Input: part model. Units: mm. Frame: model coordinates. A direction names the side the tool comes from. Coordinates: 2 decimals unless noted, no trailing zeros. Write each loop counter-clockwise with the first axis right and the second up, starting at its lowest first coordinate (ties: lowest second). Pieces come first, ordered by that corner, then holes. Notation, with made-up numbers: (79.25, 33.25) - (83.25, 33.25) arc R22 cw to (83.25, 57.25) - close; hole circle Ø11 at (16, -33). An arc over 180 degrees is marked (long way). Use a Markdown table: item, result. Add a question column.
Q1. Mould query, pull axis X, two halves, no side actions, for faces 4 (the face through (-20.63, -15.53, 2.46)), 5 (the face through (1, 36.091, 2)), 6 (the face through (-27.03, 12.79, 2.46)). Classes: released by +X, released by -X, zero draft, split by the parting line, or undercut.
Q2. Section query A-A (x = 0). Return the cut outline in (y, z).
Q3. Material intervals for probe 1 along Y at (x, z) = (0, 4); probe 2 along X at (y, z) = (-17, 2.2); probe 3 along X at (y, z) = (2.5, 2.65), sorted ascending. Write a range as from..to.
Q4. Set-up query: faces 1 (the face through (26.8, -5.44, 2.46)), 2 (the face through (19.285, -16.785, 2.465)), 3 (the face through (-27.802, -2.365, 2.465)). Return all of +Z, -Z, +X, -X, +Y, -Y with unobstructed straight access to the full face (end or side cutting, diameter ignored); none if empty.
Q5. Section query C-C (x = -10.5). Return the cut outline in (y, z), then the cut area to 3 significant figures.
Q6. Section query B-B (y = 1). Return the cut outline in (x, z), then the cut area to 3 significant figures.
Q7. Pin query (flat end, axial travel): P1, Ø1, axis at y = 4, z = 1.5, coming from the +X side; P2, Ø1.5, axis at y = -2.5, z = 2, coming from the -X side. Return the tip coordinate at first contact, or that it passes through.
Q8. Section query D-D (y = 29). Return the cut outline in (x, z), then the cut area to 3 significant figures.
from build123d import *

# Parameters (mm, degrees)
F0_R     = 8.5
F1_DEPTH = 5
F2_R     = 1
F3_R     = 1
F4_R     = 1
F5_R     = 1
F6_R     = 1
F7_R     = 1
F8_R     = 1


with BuildPart() as f1:
    # F0 (on Top) → F1 (new body)
    with BuildSketch(Plane.XY):
        with BuildLine():
            Line((-6.479281, 36.091168), (-6.720968, 28.09482))
            ThreePointArc((-6.720968, 28.09482), (-11.514328, 26.205734), (-15.818653, 23.374172))
            Line((-15.818653, 23.374172), (-22.920961, 28.017285))
            Line((-22.920961, 28.017285), (-30.745783, 15.219936))
            Line((-30.745783, 15.219936), (-24.049722, 10.842405))
            ThreePointArc((-24.049722, 10.842405), (-24.974739, 5.138761), (-24.565617, -0.624904))
            Line((-24.565617, -0.624904), (-32.038972, -4.643641))
            Line((-32.038972, -4.643641), (-24.538972, -17.634022))
            Line((-24.538972, -17.634022), (-17.493087, -13.845154))
            ThreePointArc((-17.493087, -13.845154), (-13.460411, -17.051783), (-8.856044, -19.363657))
            Line((-8.856044, -19.363657), (-9.325944, -27.835993))
            Line((-9.325944, -27.835993), (5.669297, -28.213812))
            Line((5.669297, -28.213812), (6.112319, -20.226088))
            ThreePointArc((6.112319, -20.226088), (10.95174, -18.458337), (15.326021, -15.736091))
            Line((15.326021, -15.736091), (16.301248, -14.939212))
            Line((16.301248, -14.939212), (23.187839, -19.197642))
            Line((23.187839, -19.197642), (30.453803, -7.960425))
            Line((30.453803, -7.960425), (23.870128, -3.415624))
            ThreePointArc((23.870128, -3.415624), (24.938515, 2.262912), (24.674697, 8.035054))
            Line((24.674697, 8.035054), (32.246905, 11.864276))
            Line((32.246905, 11.864276), (25.076486, 25.039446))
            Line((25.076486, 25.039446), (17.937403, 21.429252))
            ThreePointArc((17.937403, 21.429252), (13.460411, 25.082162), (8.264369, 27.609685))
            Line((8.264369, 27.609685), (8.520719, 36.091168))
            Line((8.520719, 36.091168), (-6.479281, 36.091168))
        make_face()
        with Locations((0, 4.01519)):
            Circle(F0_R, mode=Mode.SUBTRACT)
    extrude(amount=F1_DEPTH)

    # F2
    f2_edges = [f1.edges().sort_by_distance(p)[0] for p in [
        (-24.538972, -17.634022, 2.5),
        (-32.038972, -4.643641, 2.5),
    ]]
    fillet(f2_edges, radius=F2_R)

    # F3
    f3_edges = [f1.edges().sort_by_distance(p)[0] for p in [
        (-9.325944, -27.835993, 2.5),
    ]]
    fillet(f3_edges, radius=F3_R)

    # F4
    f4_edges = [f1.edges().sort_by_distance(p)[0] for p in [
        (-22.920961, 28.017285, 2.5),
    ]]
    fillet(f4_edges, radius=F4_R)

    # F5
    f5_edges = [f1.edges().sort_by_distance(p)[0] for p in [
        (-30.745783, 15.219936, 2.5),
    ]]
    fillet(f5_edges, radius=F5_R)

    # F6
    f6_edges = [f1.edges().sort_by_distance(p)[0] for p in [
        (5.669297, -28.213812, 2.5),
    ]]
    fillet(f6_edges, radius=F6_R)

    # F7
    f7_edges = [f1.edges().sort_by_distance(p)[0] for p in [
        (23.187839, -19.197642, 2.5),
        (30.453803, -7.960425, 2.5),
        (32.246905, 11.864276, 2.5),
    ]]
    fillet(f7_edges, radius=F7_R)

    # F8
    f8_edges = [f1.edges().sort_by_distance(p)[0] for p in [
        (25.076486, 25.039446, 2.5),
        (8.520719, 36.091168, 2.5),
        (-6.479281, 36.091168, 2.5),
    ]]
    fillet(f8_edges, radius=F8_R)


solid = f1.part
Values follow:
| question | item | result |
|---|---|---|
| 1 | face 4 | undercut |
| 1 | face 5 | zero draft |
| 1 | face 6 | released by -X |
| 2 | outline | (-28.07, 0) - (-4.48, 0) - (-4.48, 5) - (-28.07, 5) - close; (12.52, 0) - (36.09, 0) - (36.09, 5) - (12.52, 5) - close |
| 3 | probe 1 | -28.07..-4.48, 12.52..36.09 |
| 3 | probe 2 | -24.87..-23.36, -13.54..13.54, 19.63..24.61 |
| 3 | probe 3 | -24.95..-8.36, 8.36..24.95 |
| 4 | face 1 | +Z, -Z, +X |
| 4 | face 2 | +Z, -Z, -Y |
| 4 | face 3 | +Z, -Z, -X |
| 5 | outline | (-18.67, 0) - (26.7, 0) - (26.7, 5) - (-18.67, 5) - close |
| 5 | area | 227 mm2 |
| 6 | outline | (-24.82, 0) - (-7.95, 0) - (-7.95, 5) - (-24.82, 5) - close; (7.95, 0) - (24.82, 0) - (24.82, 5) - (7.95, 5) - close |
| 6 | area | 169 mm2 |
| 7 | P1 | x = 25 |
| 7 | P2 | x = -29.45 |
| 8 | outline | (-6.69, 0) - (8.31, 0) - (8.31, 5) - (-6.69, 5) - close |
| 8 | area | 75.0 mm2 |
